Check sheet for the drawn part. Datum: minimum x, y, z corner. Units: mm. A direction names the side the tool comes from. Coordinates: 2 decimals unless noted, no trailing zeros. Loops run counter-clockwise (first coordinate to the right, second up) from the corner with the lowest first, then second, coordinate; pieces in that order, holes last. Notation, with made-up numbers: (4, 35) - (33, 35) arc R31 cw to (33, 59) - close; hole circle Ø6 at (12.5, -30.75). An arc over 180 degrees is marked (long way). Answer as CSV lines item,"result". Start each with the question number.
1. Release check for a two-part mould opening along Y. For the marked faces 6, 7 and 8 record: pulls with the +Y half, pulls with the -Y half, needs draft (parallel to the pull), parting line crosses it, or undercut.
2. Cross-section at D-D (x = 11.75). Enter the section's corners in (y, z).
3. Cross-section at A-A (x = 25). Enter the section's corners in (y, z) (3 decimals), plus the area to 3 significant figures.
4. Cross-section at B-B (z = 1). Enter the section's corners in (x, y) (3 decimals).
5. Material ranges on line 1 (Y direction, x = 26.25, z = 1.35) (3 decimals); line 2 (X direction, y = 10, z = 0.6); line 3 (Y direction, x = 23.25, z = 0.5), recorded low to high. Write a range as [from, to].
6. Cross-section at C-C (y = 12). Enter the section's corners in (x, z).
7. Gauge pin test, flat ends, axial feed: P1, Ø2, axis at y = 11.5, z = 2.5, coming from the +X side; P2, Ø1.2, axis at x = 27.5, z = 2, coming from the -Y side (3 decimals); P3, Ø2, axis at x = 26.5, z = 3, coming from the +Y side (3 decimals). Record the tip position at first contact, or that the pin passes through.
8. Set-up check for the marked faces 1, 2, 3, 4 and 5: record each of +Z, -Z, +X, -X, +Y, -Y from which the full face is reachable in a straight line by a thin tool's end or side.
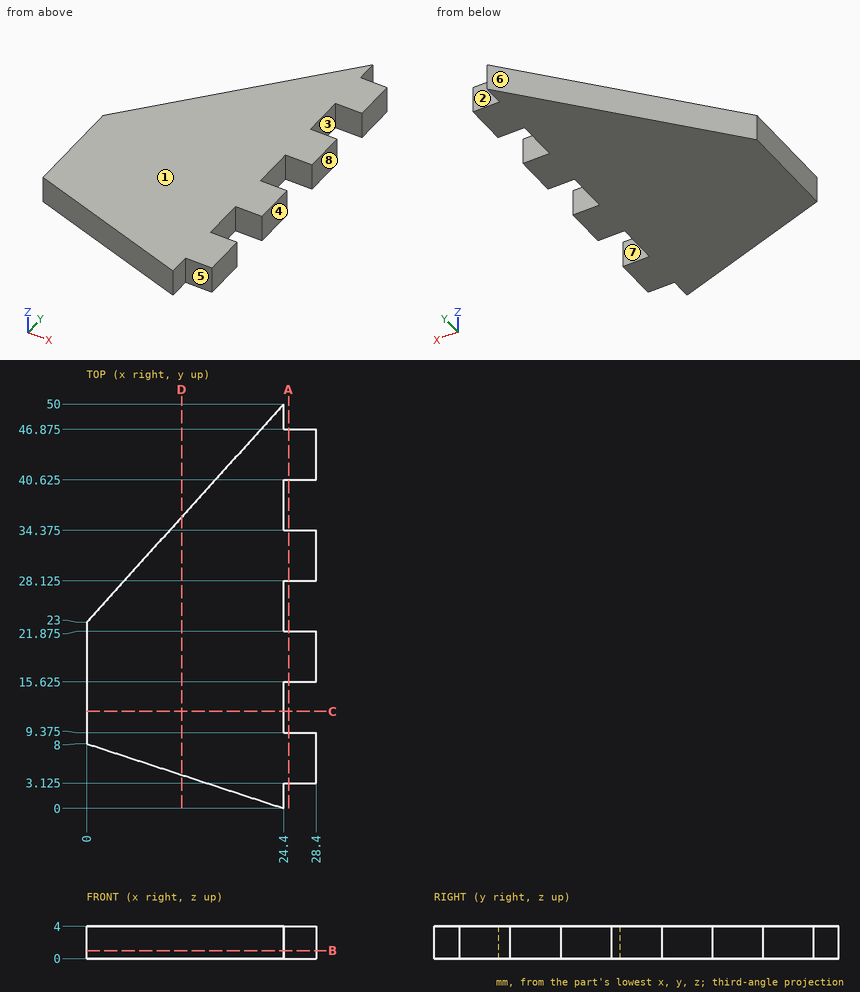
Values follow:
1,face 6,"pulls with the +Y half"
1,face 7,"undercut"
1,face 8,"needs draft"
2,outline,"(4.15, 0) - (36, 0) - (36, 4) - (4.15, 4) - close"
3,outline,"(3.125, 0) - (9.375, 0) - (9.375, 4) - (3.125, 4) - close; (15.625, 0) - (21.875, 0) - (21.875, 4) - (15.625, 4) - close; (28.125, 0) - (34.375, 0) - (34.375, 4) - (28.125, 4) - close; (40.625, 0) - (46.875, 0) - (46.875, 4) - (40.625, 4) - close"
3,area,"100 mm²"
4,outline,"(0, 8) - (24.4, 0) - (24.4, 3.125) - (28.4, 3.125) - (28.4, 9.375) - (24.4, 9.375) - (24.4, 15.625) - (28.4, 15.625) - (28.4, 21.875) - (24.4, 21.875) - (24.4, 28.125) - (28.4, 28.125) - (28.4, 34.375) - (24.4, 34.375) - (24.4, 40.625) - (28.4, 40.625) - (28.4, 46.875) - (24.4, 46.875) - (24.4, 50) - (0, 23) - close"
5,line 1,"y = [3.125, 9.375], [15.625, 21.875], [28.125, 34.375], [40.625, 46.875]"
5,line 2,"x = [0, 24.4]"
5,line 3,"y = [0.38, 48.73]"
6,outline,"(0, 0) - (24.4, 0) - (24.4, 4) - (0, 4) - close"
7,P1,"stops at x = 24.4"
7,P2,"stops at y = 3.125"
7,P3,"stops at y = 46.875"
8,face 1,"+Z, +X, -X, +Y, -Y"
8,face 2,"+Z, -Z, +X, +Y"
8,face 3,"+Z, -Z, +X"
8,face 4,"+Z, -Z, +X, +Y, -Y"
8,face 5,"+Z, -Z, +X, -Y"
